Autodesk Inventor part; units mm, degrees
ref_plane "YZ Plane" through (0, 0, 0) normal (1, 0, 0) x (0, 1, 0)
ref_plane "XZ Plane" through (0, 0, 0) normal (0, 1, 0) x (-1, 0, 0)
ref_plane "XY Plane" through (0, 0, 0) normal (0, 0, 1) x (1, 0, 0)
sketch "Эскиз1" plane through (0, 0, 0) normal (0, 1, 0) x (-1, 0, 0)
  arc A0 (11.1553, 1) -> (11.1553, -1) centre (0, 0) ccw
  line L0 (-15, 15) -> (-15, -15)
  line L1 (-15, 15) -> (0, 15)
  line L2 (-15, -15) -> (0, -15)
  line L3 (11.1553, 1) -> (14.9666, 1)
  line L4 (14.9666, -1) -> (11.1553, -1)
  arc A1 (0, -15) -> (14.5107, -3.8) centre (0, 0) ccw
  arc A2 (14.5107, 3.8) -> (0, 15) centre (0, 0) ccw
  line L5 (11.1553, -1) -> (21.1553, -1)
  line L6 (21.1553, -1) -> (21.1553, -3.8)
  line L7 (21.1553, -3.8) -> (14.5107, -3.8)
  line L8 (11.1553, 1) -> (21.1553, 1)
  line L9 (21.1553, 1) -> (21.1553, 3.8)
  line L10 (21.1553, 3.8) -> (14.5107, 3.8)
  point P0 (15, 0)
  dimension "d0" = 22.4
  dimension "d2" = 30
  dimension "d5" = 2.8
  dimension "d6" = 2.8
extrude "Выдавливание1" add sketch "Эскиз1" along normal blind 10
sketch "Эскиз2" plane through (15, 0, 15) normal (1, 0, 0) x (0, 0, -1)
  line L0 (0, 0) -> (30, 0)
  line L1 (30, 0) -> (30, 10)
  line L2 (0, 10) -> (30, 10)
  line L3 (0, 0) -> (0, 10)
  line L4 (0, 5) -> (30, 5) construction
  line L5 (15, 10) -> (15, 0) construction
  point P0 (21, 5)
  point P1 (9, 5)
  dimension "d10" = 6
  dimension "d11" = 6
hole "Отверстие1" at (15, 5, -6) at (15, 5, 6) direction (-1, 0, 0) diameter 3 depth 8 tip angle 118
fillet "Сопряжение1" radius 4 4 edges at (-21.1553, 10, 2.4) (-21.1553, 10, -2.4) (-21.1553, 0, 2.4) (-21.1553, 0, -2.4)
sketch "Эскиз3" plane through (-14.5107, 0, 3.8) normal (0, 0, 1) x (1, 0, 0)
  arc A0 (-6.6446, 4) -> (-2.6446, 0) centre (-2.6446, 4) ccw
  line L0 (-2.6446, 0) -> (0, 0)
  line L1 (0, 0) -> (0, 10)
  line L2 (-2.6446, 10) -> (0, 10)
  arc A1 (-2.6446, 10) -> (-6.6446, 6) centre (-2.6446, 6) ccw
  line L3 (-6.6446, 4) -> (-6.6446, 6)
  line L4 (-6.6446, 5) -> (-3.1446, 5) construction
  point P0 (14.5107, 0)
  dimension "d20" = 3.5
hole "Отверстие2" at (-17.6553, 5, 3.8) direction (0, 0, -1) diameter 3 depth 8 tip angle 118
fillet "Сопряжение2" radius 2 2 edges at (15, 5, 15) (15, 5, -15)
chamfer "Фаска1" distance 1 angle 45 16 edges at (11.2, 10, 0) (11.2, 0, 0) (6.5, 10, 15) (14.4142, 10, 14.4142) (15, 10, 0) (14.4142, 10, -14.4142) (6.5, 10, -15) (-9.1652, 10, -11.8743) (-9.1652, 10, 11.8743) (6.5, 0, 15) (14.4142, 0, 14.4142) (15, 0, 0) (14.4142, 0, -14.4142) (6.5, 0, -15) (-9.1652, 0, -11.8743) (-9.1652, 0, 11.8743)
properties part number "ScreenMount"
Build history of the part. All positions in model axes, mm. A direction names the side the tool comes from. Give positions to 0.01 mm unless a question says otherwise; leave off trailing zeros. Loops run counter-clockwise (first coordinate to the right, second up) from the corner with the lowest first, then second, coordinate; pieces in that order, holes last.
1) Probe line 1 along Y through (x, z) = (12.5, 6); line 2 along Z through (x, y) = (-15, 1.75); line 3 along Z through (x, y) = (0, 5.25). List the from-to ranges inside material, lowest first.
Values follow:
line 1: y = 0 to 3.5, 6.5 to 10
line 2: z = -3.8 to -1, 1 to 3.8
line 3: z = -15 to -11.2, 11.2 to 15
2) Drop flat-ended pins along their axis: P1, Ø1.8, axis at y = 5, z = -6, coming from the -X side; P2, Ø3, axis at x = -2, y = 4.5, coming from the +Z side; P3, Ø3, axis at x = -9.5, y = 8.5, coming from the -Z side. Give the stop position or say it passes through.
Values follow:
P1: stops at x = -14.11
P2: stops at z = 14.99
P3: stops at z = -12.69
3) Band-saw the part on B-B on z = 0. List the corners of the cut face in (x, y).
Values follow:
outline: (11.2, 1) - (12.2, 0) - (14, 0) - (15, 1) - (15, 9) - (14, 10) - (12.2, 10) - (11.2, 9) - close
4) Band-saw the part on A-A on y = 5. State how many separate pieces and enclosed holes the cut face has, then the cut area to 3 significant figures.
Values follow:
separate pieces: 5
enclosed holes: 0
area: 385 mm2
5) Band-saw the part on D-D on y = 7. List the corners of the cut face in (x, z), then the cut area to 3 significant figures.
Values follow:
outline: (-21.03, -3.8) - (-14.51, -3.8) arc R15 ccw to (0, -15) - (13, -15) arc R2 ccw to (15, -13) - (15, 13) arc R2 ccw to (13, 15) - (0, 15) arc R15 ccw to (-14.51, 3.8) - (-21.03, 3.8) - (-21.03, 1) - (-11.16, 1) arc R11.2 cw (long way) to (-11.16, -1) - (-21.03, -1) - close
area: 435 mm2
6) Two-plate mould, pull along Z, no slides. Class faces 1 (the face through (-9, 5, 12)), 2 (the face through (11.36, 9.17, 0.49)), 3 (the face through (6.6, 9.5, -14.5)): released by +Z, released by -Z, zero draft, split by the parting line, or undercut.
Values follow:
face 1: released by +Z
face 2: undercut
face 3: released by -Z
7) 3-axis set-ups, long thin cutter, end or side, ignore diameter. For faces 4 (the face through (-15, 5, -1)), 5 (the face through (15, 5, 0)): which of +Z, -Z, +X, -X, +Y, -Y reach the whole face in a straight line?
Values follow:
face 4: -X, +Y, -Y
face 5: +Z, -Z, +X, +Y, -Y
